Autodesk Inventor part; units mm, degrees
ref_plane "YZ Plane" through (0, 0, 0) normal (1, 0, 0) x (0, 1, 0)
ref_plane "XZ Plane" through (0, 0, 0) normal (0, 1, 0) x (-1, 0, 0)
ref_plane "XY Plane" through (0, 0, 0) normal (0, 0, 1) x (1, 0, 0)
sketch "Sketch1" plane through (0, 0, 0) normal (0, 0, 1) x (1, 0, 0)
  point P0 (0, 0)
sketch "0" plane through (0, 0, 0) normal (0, 0, 1) x (1, 0, 0)
  line L0 (7.6759, 72.8464) -> (20.6759, 72.8464)
  line L1 (7.6759, 58.8464) -> (20.6759, 58.8464)
  line L2 (7.1759, 72.3464) -> (7.1759, 59.3464)
  line L3 (21.1759, 72.3464) -> (21.1759, 59.3464)
  arc A0 (7.6759, 72.8464) -> (7.1759, 72.3464) centre (7.6759, 72.3464) ccw
  arc A1 (21.1759, 72.3464) -> (20.6759, 72.8464) centre (20.6759, 72.3464) ccw
  arc A2 (7.1759, 59.3464) -> (7.6759, 58.8464) centre (7.6759, 59.3464) ccw
  arc A3 (20.6759, 58.8464) -> (21.1759, 59.3464) centre (20.6759, 59.3464) ccw
  line L4 (26.7259, 72.8464) -> (39.7259, 72.8464)
  line L5 (26.7259, 58.8464) -> (39.7259, 58.8464)
  line L6 (26.2259, 72.3464) -> (26.2259, 59.3464)
  line L7 (40.2259, 72.3464) -> (40.2259, 59.3464)
  arc A4 (26.7259, 72.8464) -> (26.2259, 72.3464) centre (26.7259, 72.3464) ccw
  arc A5 (40.2259, 72.3464) -> (39.7259, 72.8464) centre (39.7259, 72.3464) ccw
  arc A6 (26.2259, 59.3464) -> (26.7259, 58.8464) centre (26.7259, 59.3464) ccw
  arc A7 (39.7259, 58.8464) -> (40.2259, 59.3464) centre (39.7259, 59.3464) ccw
  line L8 (45.7759, 72.8464) -> (58.7759, 72.8464)
  line L9 (45.7759, 58.8464) -> (58.7759, 58.8464)
  line L10 (45.2759, 72.3464) -> (45.2759, 59.3464)
  line L11 (59.2759, 72.3464) -> (59.2759, 59.3464)
  arc A8 (45.7759, 72.8464) -> (45.2759, 72.3464) centre (45.7759, 72.3464) ccw
  arc A9 (59.2759, 72.3464) -> (58.7759, 72.8464) centre (58.7759, 72.3464) ccw
  arc A10 (45.2759, 59.3464) -> (45.7759, 58.8464) centre (45.7759, 59.3464) ccw
  arc A11 (58.7759, 58.8464) -> (59.2759, 59.3464) centre (58.7759, 59.3464) ccw
  line L12 (7.6759, 53.7964) -> (20.6759, 53.7964)
  line L13 (7.6759, 39.7964) -> (20.6759, 39.7964)
  line L14 (7.1759, 53.2964) -> (7.1759, 40.2964)
  line L15 (21.1759, 53.2964) -> (21.1759, 40.2964)
  arc A12 (7.6759, 53.7964) -> (7.1759, 53.2964) centre (7.6759, 53.2964) ccw
  arc A13 (21.1759, 53.2964) -> (20.6759, 53.7964) centre (20.6759, 53.2964) ccw
  arc A14 (7.1759, 40.2964) -> (7.6759, 39.7964) centre (7.6759, 40.2964) ccw
  arc A15 (20.6759, 39.7964) -> (21.1759, 40.2964) centre (20.6759, 40.2964) ccw
  line L16 (26.7259, 53.7964) -> (39.7259, 53.7964)
  line L17 (26.7259, 39.7964) -> (39.7259, 39.7964)
  line L18 (26.2259, 53.2964) -> (26.2259, 40.2964)
  line L19 (40.2259, 53.2964) -> (40.2259, 40.2964)
  arc A16 (26.7259, 53.7964) -> (26.2259, 53.2964) centre (26.7259, 53.2964) ccw
  arc A17 (40.2259, 53.2964) -> (39.7259, 53.7964) centre (39.7259, 53.2964) ccw
  arc A18 (26.2259, 40.2964) -> (26.7259, 39.7964) centre (26.7259, 40.2964) ccw
  arc A19 (39.7259, 39.7964) -> (40.2259, 40.2964) centre (39.7259, 40.2964) ccw
  line L20 (45.7759, 53.7964) -> (58.7759, 53.7964)
  line L21 (45.7759, 39.7964) -> (58.7759, 39.7964)
  line L22 (45.2759, 53.2964) -> (45.2759, 40.2964)
  line L23 (59.2759, 53.2964) -> (59.2759, 40.2964)
  arc A20 (45.7759, 53.7964) -> (45.2759, 53.2964) centre (45.7759, 53.2964) ccw
  arc A21 (59.2759, 53.2964) -> (58.7759, 53.7964) centre (58.7759, 53.2964) ccw
  arc A22 (45.2759, 40.2964) -> (45.7759, 39.7964) centre (45.7759, 40.2964) ccw
  arc A23 (58.7759, 39.7964) -> (59.2759, 40.2964) centre (58.7759, 40.2964) ccw
  line L24 (-8.7991, 8.4184) -> (126.2009, 8.4184)
  line L25 (126.2009, 8.4184) -> (126.2009, 88.4184)
  line L26 (126.2009, 88.4184) -> (-8.7991, 88.4184)
  line L27 (-8.7991, 88.4184) -> (-8.7991, 8.4184)
  line L28 (66.9509, 88.4184) -> (85.4509, 88.4184)
  line L29 (85.4509, 88.4184) -> (85.4509, 57.4184)
  line L30 (85.4509, 57.4184) -> (66.9509, 57.4184)
  line L31 (66.9509, 57.4184) -> (66.9509, 88.4184)
  circle A24 centre (-3.7991, 83.4184) radius 1.7
  circle A25 centre (121.2009, 83.4184) radius 1.7
  circle A26 centre (121.2009, 13.4184) radius 1.7
  circle A27 centre (-3.7991, 13.4184) radius 1.7
  dimension "d2" = 135
  dimension "d3" = 80
  dimension "d4" = 15.975
  dimension "d5" = 15.572
  dimension "d6" = 18.5
  dimension "d7" = 31
  dimension "d8" = 75.75
  dimension "d9" = 3.4
  dimension "d10" = 3.4
  dimension "d11" = 3.4
  dimension "d12" = 3.4
  dimension "d13" = 5
  dimension "d14" = 5
  dimension "d15" = 5
  dimension "d16" = 5
  dimension "d17" = 5
  dimension "d18" = 5
  dimension "d19" = 5
  dimension "d20" = 5
extrude "Extrusion1" add sketch "0" along normal blind 1.5 contours L27 L26 L31 L30 L29 L25 L24
sketch "Sketch4" plane through (0, 0, 1.5) normal (0, 0, 1) x (1, 0, 0)
  line L0 (0.7009, 78.9184) -> (116.7009, 78.9184)
  line L1 (116.7009, 78.9184) -> (116.7009, 17.9184)
  line L2 (116.7009, 17.9184) -> (0.7009, 17.9184)
  line L3 (0.7009, 17.9184) -> (0.7009, 78.9184)
  line L4 (66.9509, 88.4184) -> (-8.7991, 88.4184)
  line L5 (126.2009, 8.4184) -> (126.2009, 88.4184)
  line L6 (-8.7991, 8.4184) -> (126.2009, 8.4184)
  line L7 (-8.7991, 88.4184) -> (-8.7991, 8.4184)
  line L8 (66.7009, 52.0684) -> (106.7009, 52.0684)
  line L9 (106.7009, 52.0684) -> (106.7009, 21.3184)
  line L10 (106.7009, 21.3184) -> (66.7009, 21.3184)
  line L11 (66.7009, 21.3184) -> (66.7009, 52.0684)
  line L12 (85.4509, 57.4184) -> (66.9509, 57.4184)
  point P0 (0, 0)
  dimension "d23" = 9.5
  dimension "d24" = 9.5
  dimension "d25" = 9.5
  dimension "d26" = 9.5
  dimension "d27" = 5.35
  dimension "d28" = 30.75
  dimension "d29" = 40
  dimension "d30" = 10
extrude "Extrusion2" cut sketch "Sketch4" against normal blind 1.5 contours L8 L9 L10 L11
sketch "Sketch5" plane through (0, 0, 1.5) normal (0, 0, 1) x (1, 0, 0)
  line L0 (1.9509, 29.1684) -> (62.9509, 29.1684)
  line L1 (62.9509, 29.1684) -> (62.9509, 19.1684)
  line L2 (62.9509, 19.1684) -> (1.9509, 19.1684)
  line L3 (1.9509, 19.1684) -> (1.9509, 29.1684)
  line L4 (-8.7991, 8.4184) -> (126.2009, 8.4184)
  line L5 (-8.7991, 88.4184) -> (-8.7991, 8.4184)
  point P0 (0, 0)
  dimension "d33" = 61
  dimension "d34" = 10
  dimension "d35" = 10.75
  dimension "d36" = 10.75
extrude "Extrusion3" cut sketch "Sketch5" against normal blind 1.5
fillet "Fillet1" radius 5 4 edges at (-8.7991, 8.4184, 0.75) (-8.7991, 88.4184, 0.75) (126.2009, 88.4184, 0.75) (126.2009, 8.4184, 0.75)
properties part number "Top_Case"
Verification items for the finished model (mm, model axes). Give positions to 0.01 mm unless a question says otherwise; leave off trailing zeros. Loops run counter-clockwise (first coordinate to the right, second up) from the corner with the lowest first, then second, coordinate; pieces in that order, holes last. Notation, with made-up numbers: M 85.5,-16 L 127.5,-16 A15 cw 127.5,5 Z; hole C -4.5,-10 d1. An arc over 180 degrees is marked long. Return JSON: item names as keys, results as strings.
1) Section check C-C, the plane z = 0.8. Count the separate pieces of the cut face and the enclosed holes in it, and give its area (3 significant figures).
Findings:
{"separate pieces": "1", "enclosed holes": "12", "area": "7,150 mm2"}
2) Material ranges on L1, parallel to X at y = 49, z = 1.2; L2, parallel to X at y = 67, z = 1; L3, parallel to Y at x = 34, z = 1.2, recorded low to high. Write a range as [from, to].
Findings:
{"L1": "x = [-8.8, 7.18], [21.18, 26.23], [40.23, 45.28], [59.28, 66.7], [106.7, 126.2]", "L2": "x = [-8.8, 7.18], [21.18, 26.23], [40.23, 45.28], [59.28, 66.95], [85.45, 126.2]", "L3": "y = [8.42, 19.17], [29.17, 39.8], [53.8, 58.85], [72.85, 88.42]"}
3) Mould release check, pull along Y, two halves, no side actions. Record for faces 1 (the cylindrical face through (122.822, 12.908, 0.74)), 2 (the flat face through (58, 58, 1.5)), 3 (the cylindrical face through (124.697, 9.844, 0.76)): released by +Y, released by -Y, zero draft, split by the parting line, or undercut.
Findings:
{"face 1": "undercut", "face 2": "zero draft", "face 3": "released by -Y"}
4) Section check A-A, the plane x = 23. Enter the section's corners in (y, z), and give its area (3 significant figures).
Findings:
{"outline": "M 8.42,0 L 19.17,0 L 19.17,1.5 L 8.42,1.5 Z; M 29.17,0 L 88.42,0 L 88.42,1.5 L 29.17,1.5 Z", "area": "105 mm2"}
5) Gauge pin test, flat end, axial feed: P1, Ø3, axis at x = 121.2, y = 13.42, coming from the +Z side. Record the tip position at first contact, or that the pin passes through.
Findings:
{"P1": "passes through"}
6) Section check B-B, the plane y = 78.5. Enter the section's corners in (x, z), and give its area (3 significant figures).
Findings:
{"outline": "M -8.8,0 L 66.95,0 L 66.95,1.5 L -8.8,1.5 Z; M 85.45,0 L 126.2,0 L 126.2,1.5 L 85.45,1.5 Z", "area": "175 mm2"}
